```python
from build123d import *

# Parameters (mm, degrees)
BOSS_EXTRU_1_DEPTH      = 3
D_GAGEMENT_M42_D        = 4.5
D_GAGEMENT_M42_DEPTH    = 10
D_GAGEMENT_M42_TIP      = 1.351936393
D_GAGEMENT_M221_D       = 24
D_GAGEMENT_M221_DEPTH   = 10
D_GAGEMENT_M221_TIP     = 7.210327428
D_GAGEMENT_M121_D       = 13.5
D_GAGEMENT_M121_DEPTH   = 10
D_GAGEMENT_M121_TIP     = 4.055809178
D_GAGEMENT_M101_D       = 11
D_GAGEMENT_M101_DEPTH   = 10
D_GAGEMENT_M101_TIP     = 3.304733405
ESQUISSE26_W            = 27.5
ESQUISSE26_H            = 21
ENL_V_MAT_EXTRU_1_DEPTH = 10
D_GAGEMENT_M31_D        = 3.4
D_GAGEMENT_M201_D       = 22
D_GAGEMENT_M33_D        = 3.4


with BuildPart() as part:
    # Esquisse1 → Boss.-Extru.1 (new body)
    with BuildSketch(Plane.XY):
        with BuildLine():
            Line((-145, 85), (-109.886246, 120.113754))
            Line((-109.886246, 120.113754), (109.886246, 120.113754))
            Line((109.886246, 120.113754), (145, 85))
            Line((145, 85), (145, -85))
            Line((145, -85), (109.886246, -120.113754))
            Line((109.886246, -120.113754), (104.886246, -120.113754))
            ThreePointArc((104.886246, -120.113754), (0, -20), (-104.886246, -120.113754))
            Line((-104.886246, -120.113754), (-109.886246, -120.113754))
            Line((-109.886246, -120.113754), (-145, -85))
            Line((-145, -85), (-145, 85))
        make_face()
    extrude(amount=BOSS_EXTRU_1_DEPTH)

    # Dégagement M42
    with Locations(Plane.XY.offset(3)):
        with Locations((-139.3, 79.3), (-139.3, -79.3), (139.3, -79.3), (139.3, 79.3)):
            Hole(D_GAGEMENT_M42_D / 2, depth=D_GAGEMENT_M42_DEPTH)
            with Locations((0, 0, -(D_GAGEMENT_M42_DEPTH + D_GAGEMENT_M42_TIP / 2))):  # 118° drill point
                Cone(0, D_GAGEMENT_M42_D / 2, D_GAGEMENT_M42_TIP, mode=Mode.SUBTRACT)

    # Dégagement M221
    with Locations(Plane.XY.offset(3)):
        with Locations((-100, 75.113754)):
            Hole(D_GAGEMENT_M221_D / 2, depth=D_GAGEMENT_M221_DEPTH)
            with Locations((0, 0, -(D_GAGEMENT_M221_DEPTH + D_GAGEMENT_M221_TIP / 2))):  # 118° drill point
                Cone(0, D_GAGEMENT_M221_D / 2, D_GAGEMENT_M221_TIP, mode=Mode.SUBTRACT)

    # Dégagement M121
    with Locations(Plane.XY.offset(3)):
        with Locations((100, 75.113754), (100, 45.113754)):
            Hole(D_GAGEMENT_M121_D / 2, depth=D_GAGEMENT_M121_DEPTH)
            with Locations((0, 0, -(D_GAGEMENT_M121_DEPTH + D_GAGEMENT_M121_TIP / 2))):  # 118° drill point
                Cone(0, D_GAGEMENT_M121_D / 2, D_GAGEMENT_M121_TIP, mode=Mode.SUBTRACT)

    # Dégagement M101
    with Locations(Plane.XY.offset(3)):
        with Locations((-38.75, 75.113754), (38.75, 75.113754)):
            Hole(D_GAGEMENT_M101_D / 2, depth=D_GAGEMENT_M101_DEPTH)
            with Locations((0, 0, -(D_GAGEMENT_M101_DEPTH + D_GAGEMENT_M101_TIP / 2))):  # 118° drill point
                Cone(0, D_GAGEMENT_M101_D / 2, D_GAGEMENT_M101_TIP, mode=Mode.SUBTRACT)

    # Esquisse26 → Enlèv. mat.-Extru.1 (cut)
    with BuildSketch(Plane.XY.offset(3)):
        with Locations((0, 75.113754)):
            Rectangle(ESQUISSE26_W, ESQUISSE26_H)
    extrude(amount=-ENL_V_MAT_EXTRU_1_DEPTH, mode=Mode.SUBTRACT)

    # Dégagement M31 (through all)
    with Locations(Plane.XY.offset(3)):
        with Locations((0, 111.413754), (-90, 111.413754), (90, 111.413754)):
            Hole(D_GAGEMENT_M31_D / 2)

    # Dégagement M201 (through all)
    with Locations(Plane.XY.offset(3)):
        with Locations((0, 10.113754)):
            Hole(D_GAGEMENT_M201_D / 2)

    # Dégagement M33 (through all)
    with Locations(Plane.XY.offset(3)):
        with Locations((-20, 30.113754), (20, 30.113754), (20, -9.886246), (-20, -9.886246)):
            Hole(D_GAGEMENT_M33_D / 2)


solid = part.part
```
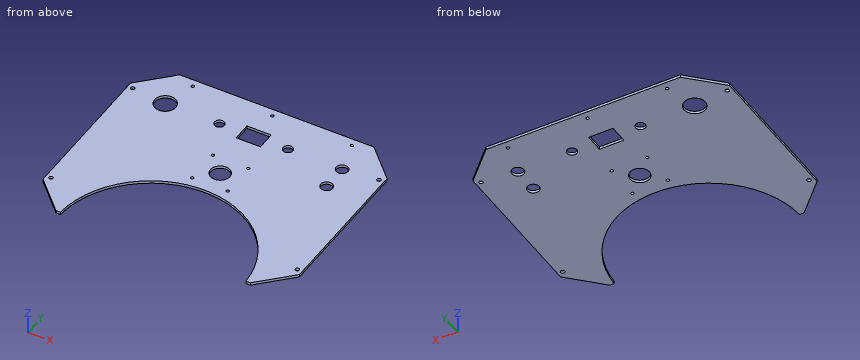
The listing builds one solid part. Answer for the finished solid, in the listing's coordinates (mm). Give positions to 0.01 mm unless a question says otherwise; leave off trailing zeros. Order: outer loops, then holes, each group sorted by start corner. A loop starts at its lowest first (then second) coordinate and runs counter-clockwise, first axis right, second up. Notation, with made-up numbers: (11.25, 35.5) - (31.25, 35.5) arc R30 ccw to (31.25, 72.5) - close; hole circle Ø6 at (8, 19.25). An arc over 180 degrees is marked (long way). Use one line per item in the form item = value. Start each with the question number.
(1) A flat-ended cylindrical pin translates along its axis: pin 1 Ø2.5 at (x, y) = (139.3, -79.3) entering from -Z (1 decimal). Find the tip coordinate at first contact, or state that the pin passes through.
(2) Consider line 1 (Y direction, x = 94.5, z = 1.3); line 2 (Y direction, x = -139.3, z = 1.3); line 3 (X direction, y = 67, z = 0.75). Determine where each line is inside the solid, lowest interval first. Write a range as from..to.
(3) A cutting plane is placed at A-A, the plane x = 100. Write down the section's boundary in (y, z).
(4) A cutting plane is placed at C-C, the plane x = -100. Write down the section's boundary in (y, z).
(5) A cutting plane is placed at B-B, the plane z = 1.65. State how many separate pieces and enclosed holes the cut face has, then the cut area to 3 significant figures.
Ans:
q1.pin_1 = through
q2.line_1 = -79.23..41.2, 49.03..71.2, 79.03..120.11
q2.line_2 = -90.7..-81.55, -77.05..77.05, 81.55..90.7
q2.line_3 = -145..-108.84, -91.16..-13.75, 13.75..145
q3.outline = (-92.98, 0) - (38.36, 0) - (38.36, 3) - (-92.98, 3) - close; (51.86, 0) - (68.36, 0) - (68.36, 3) - (51.86, 3) - close; (81.86, 0) - (120.11, 0) - (120.11, 3) - (81.86, 3) - close
q4.outline = (-92.98, 0) - (63.11, 0) - (63.11, 3) - (-92.98, 3) - close; (87.11, 0) - (120.11, 0) - (120.11, 3) - (87.11, 3) - close
q5.separate_pieces = 1
q5.enclosed_holes = 18
q5.area = 48,900 mm^2
